```python
from build123d import *

# Parameters (mm, degrees)
F0_W     = 30
F0_H     = 30
F1_DEPTH = 3
F2_R     = 1
F3_W     = 26
F3_H     = 26
F4_DEPTH = 20
F5_R     = 2
F6_W     = 22
F6_H     = 22
F7_DEPTH = 20


with BuildPart() as f1:
    # F0 (on Top) → F1 (new body)
    with BuildSketch(Plane.XY):
        Rectangle(F0_W, F0_H)
    extrude(amount=F1_DEPTH)

    # F2
    f2_edges = [f1.edges().sort_by_distance(p)[0] for p in [
        (-15, 15, 1.5),
        (-15, -15, 1.5),
        (15, -15, 1.5),
        (15, 15, 1.5),
    ]]
    fillet(f2_edges, radius=F2_R)

    # F3 (on face) → F4 (join)
    with BuildSketch(Plane.XY.offset(3)):
        Rectangle(F3_W, F3_H)
    extrude(amount=F4_DEPTH)

    # F5
    f5_edges = [f1.edges().sort_by_distance(p)[0] for p in [
        (-13, -13, 13),
        (13, -13, 13),
        (13, 13, 13),
        (-13, 13, 13),
    ]]
    fillet(f5_edges, radius=F5_R)

    # F6 (on face) → F7 (cut, through all)
    with BuildSketch(Plane.XY.offset(23)):
        Rectangle(F6_W, F6_H)
    extrude(amount=-F7_DEPTH, mode=Mode.SUBTRACT)


solid = f1.part
```
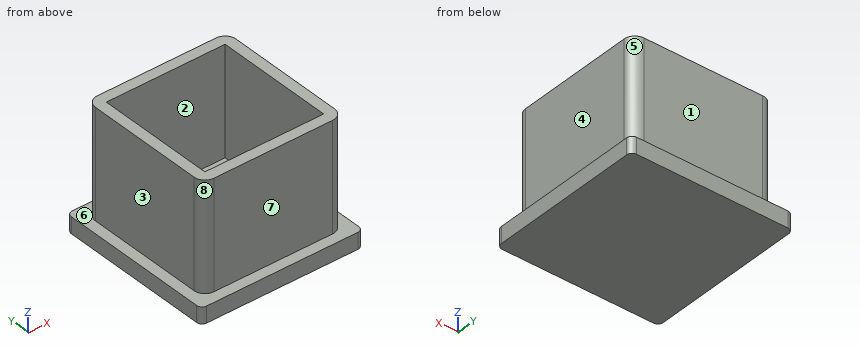
Part model, mm, in its own coordinate system. Face numbers are marked on the shaded views. A direction names the side the tool comes from. Round coordinates to 2 decimals unless told otherwise and drop trailing zeros. Loops run counter-clockwise (first coordinate to the right, second up) from the corner with the lowest first, then second, coordinate; pieces in that order, holes last.
Item 1: 3-axis set-ups, long thin cutter, end or side, ignore diameter. For the marked faces 4, 5, 6, 7 and 8: which of +Z, -Z, +X, -X, +Y, -Y reach the whole face in a straight line?
Item 2: Drop flat-ended pins along their axis: P1, Ø2, axis at x = 1.5, z = 15.5, coming from the +Y side; P2, Ø12, axis at y = -4.5, z = 9.5, coming from the +X side; P3, Ø6.5, axis at x = -0.5, y = -2, coming from the +Z side. Give the stop position or say it passes through.
Item 3: Mould opens along Y. For the marked faces 1, 2 and 3 say: +Y half, -Y half, draft (parallel to the pull), parting line (faces both ways), or undercut.
Item 4: Cut at B-B, the plane y = 9.5. Give the cut face in (x, z).
Item 5: Cut at A-A, the plane z = 6.5. Give the cut face in (x, y), then the cut area to 3 significant figures.
Item 6: Drill centre lines: line 1 (Y direction, x = 9, z = 17.5); line 2 (Z direction, x = -2.25, y = 0.75). Where is each one in solid material? Low to high.
A:
1. face 4: +Z, +X, +Y, -Y
1. face 5: +Z, +X, +Y
1. face 6: +Z
1. face 7: +Z, +X, -X, -Y
1. face 8: +Z, -X, -Y
2. P1: stops at y = 13
2. P2: stops at x = 13
2. P3: stops at z = 3
3. face 1: +Y half
3. face 2: undercut
3. face 3: draft
4. outline: (-15, 0) - (15, 0) - (15, 3) - (13, 3) - (13, 23) - (11, 23) - (11, 3) - (-11, 3) - (-11, 23) - (-13, 23) - (-13, 3) - (-15, 3) - close
5. outline: (-13, -11) arc R2 ccw to (-11, -13) - (11, -13) arc R2 ccw to (13, -11) - (13, 11) arc R2 ccw to (11, 13) - (-11, 13) arc R2 ccw to (-13, 11) - close; hole (-11, -11) - (11, -11) - (11, 11) - (-11, 11) - close
5. area: 189 mm2
6. line 1: y = -13 to -11, 11 to 13
6. line 2: z = 0 to 3
